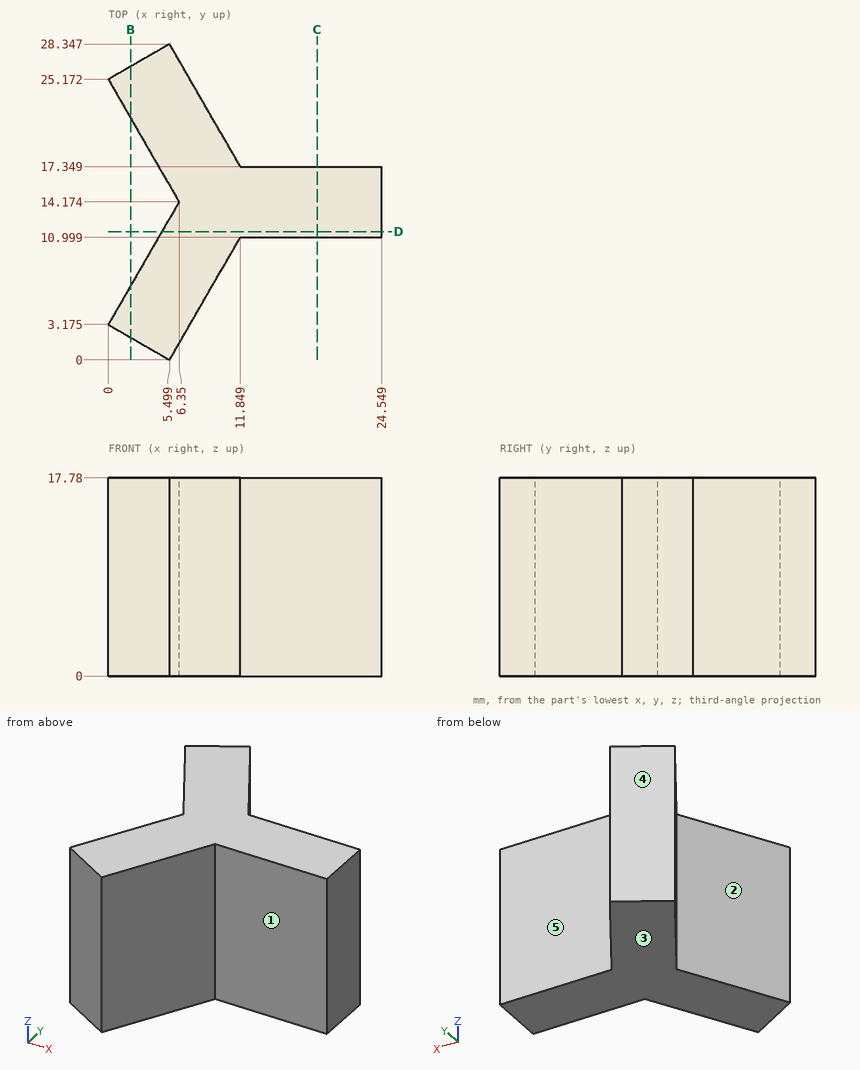
Could you check a few things on this drawing? It's one solid part, dimensions in mm from its lowest x, y, z. A direction names the side the tool comes from. Give positions to 0.01 mm unless a question says otherwise; leave off trailing zeros. Loops run counter-clockwise (first coordinate to the right, second up) from the corner with the lowest first, then second, coordinate; pieces in that order, holes last. Notation, with made-up numbers: M -7.5,34 L 48.5,34 A21 cw 48.5,66 Z; hole C -2.75,68.25 d8. An arc over 180 degrees is marked long. Answer as a JSON object with one key per item and string values.
Q1. Suppose I cut it at B-B, the plane x = 2. List the corners of the cut face in (y, z) for me.
Values found:
{"outline": "M 2.02,0 L 6.64,0 L 6.64,17.78 L 2.02,17.78 Z; M 21.71,0 L 26.33,0 L 26.33,17.78 L 21.71,17.78 Z"}
Q2. Suppose I cut it at C-C, the plane x = 18.75. List the corners of the cut face in (y, z) for me, plus the area to 3 significant figures.
Values found:
{"outline": "M 11,0 L 17.35,0 L 17.35,17.78 L 11,17.78 Z", "area": "113 mm²"}
Q3. For P1, Ø1, axis at y = 16.5, z = 9, coming from the -X side; P2, Ø10, axis at x = 20.5, z = 4.5, coming from the +Y side; P3, Ø3, axis at x = 7.5, y = 19, coming from the -Z side; P4, Ø2, axis at y = 22, z = 4, coming from the -X side (1 decimal), each with a flat end and sliding along its axis, tell me the tip position at first contact or that it passes through.
Values found:
{"P1": "stops at x = 4.72", "P2": "stops at y = 17.35", "P3": "stops at z = 0", "P4": "stops at x = 1.3"}
Q4. Suppose I cut it at D-D, the plane y = 11.5. List the corners of the cut face in (x, z) for me, plus the area to 3 significant figures.
Values found:
{"outline": "M 4.81,0 L 24.55,0 L 24.55,17.78 L 4.81,17.78 Z", "area": "351 mm²"}
Q5. If I drill on probe 1 along Y at (x, z) = (13, 4.25); probe 2 along Y at (x, z) = (3, 1.5) (1 decimal); probe 3 along Y at (x, z) = (5.75, 7.75) (1 decimal), over which ranges is the centre line in solid material (lowest first)? Write a range as [from, to].
Values found:
{"probe 1": "y = [11, 17.35]", "probe 2": "y = [1.4, 8.4], [20, 26.9]", "probe 3": "y = [0.4, 13.1], [15.2, 27.9]"}
Q6. For the marked faces 1, 2, 3, 4 and 5, which set-ups out of +Z, -Z, +X, -X, +Y, -Y let a thin tool reach every point of the face, with its end or its side?
Values found:
{"face 1": "+Z, -Z, +X, -Y", "face 2": "+Z, -Z, -X", "face 3": "-Z, +X, -X, +Y, -Y", "face 4": "+Z, -Z, -X, +Y", "face 5": "+Z, -Z, +X, +Y"}
